from build123d import *

# Parameters (mm, degrees)
BOSS_EXTRUDE1_DEPTH = 3
BOSS_EXTRUDE2_DEPTH = 3
BOSS_EXTRUDE3_DEPTH = 30
FILLET1_R           = 3
CUT_EXTRUDE1_REACH  = 120.494
SKETCH6_R           = 7.5
CUT_EXTRUDE2_REACH  = 120.494
SKETCH7_W           = 30
SKETCH7_H           = 10
CUT_EXTRUDE3_START  = -36
SKETCH8_R           = 2.1
CUT_EXTRUDE3_DEPTH  = 36
FILLET2_R           = 1


with BuildPart() as part:
    # Sketch2 → Boss-Extrude1 (new body)
    with BuildSketch(Plane.XY):
        Polygon((165.715003736, 148.457007378), (35.636413421, 16.910208322), (54.124071667, -1.371107074), (184.202661981, 130.175691982), align=None)
    extrude(amount=-BOSS_EXTRUDE1_DEPTH)



with BuildPart() as body_2:
    # Sketch4 → Boss-Extrude2 (new body)
    with BuildSketch(Plane(origin=(0, 0, -36), x_dir=(-1, 0, 0), z_dir=(0, 0, -1))):
        Polygon((-165.715003736, 148.457007378), (-184.202661981, 130.175691982), (-54.124071667, -1.371107074), (-35.636413421, 16.910208322), align=None)
    extrude(amount=-BOSS_EXTRUDE2_DEPTH)


with BuildPart() as part_1:
    add(part.part)

    add(body_2.part)  # Boss-Extrude3 merges body 2
    # Sketch5 → Boss-Extrude3 (add)
    with BuildSketch(Plane(origin=(0, 0, -3), x_dir=(-1, 0, 0), z_dir=(0, 0, -1))):
        Polygon((-35.636413421, 16.910208322), (-165.715003736, 148.457007378), (-167.848195072, 146.347624832), (-37.769604757, 14.800825776), align=None)
    extrude(amount=BOSS_EXTRUDE3_DEPTH)

    # Fillet1
    fillet1_edges = [part_1.edges().sort_by_distance(p)[0] for p in [
        (100.675708579, 82.68360785, -36),
        (102.808899915, 80.574225304, -33),
        (102.808899915, 80.574225304, -3),
        (100.675708579, 82.68360785, 0),
    ]]
    fillet(fillet1_edges, radius=FILLET1_R)

    # Sketch6 → Cut-Extrude1 (cut, up to next)
    with BuildSketch(Plane(origin=(9.563615855, -9.456875254, 0), x_dir=(0, 0, 1), z_dir=(-0.711063779, 0.703127515, 0)), mode=Mode.PRIVATE) as cut_extrude1_sk1:
        with Locations((-18, 197.081179448)):
            Circle(SKETCH6_R)
    cut_extrude1_tool1 = extrude(cut_extrude1_sk1.sketch, amount=-CUT_EXTRUDE1_REACH, mode=Mode.PRIVATE) & part_1.part
    add(cut_extrude1_tool1.solids().sort_by_distance((148.136816, 130.680413, -18))[0], mode=Mode.SUBTRACT)

    # Sketch7 → Cut-Extrude2 (cut, up to next)
    with BuildSketch(Plane(origin=(9.563615855, -9.456875254, 0), x_dir=(0, 0, 1), z_dir=(-0.711063779, 0.703127515, 0)), mode=Mode.PRIVATE) as cut_extrude2_sk1:
        with Locations((-18, 217.081179448)):
            Rectangle(SKETCH7_W, SKETCH7_H)
    cut_extrude2_tool1 = extrude(cut_extrude2_sk1.sketch, amount=-CUT_EXTRUDE2_REACH, mode=Mode.PRIVATE) & part_1.part
    add(cut_extrude2_tool1.solids().sort_by_distance((162.199366, 144.901688, -18))[0], mode=Mode.SUBTRACT)
    # Sketch7 → Cut-Extrude2 (cut, up to next)
    with BuildSketch(Plane(origin=(9.563615855, -9.456875254, 0), x_dir=(0, 0, 1), z_dir=(-0.711063779, 0.703127515, 0)), mode=Mode.PRIVATE) as cut_extrude2_sk2:
        with Locations((-18, 42.081179448)):
            Rectangle(SKETCH7_W, SKETCH7_H)
    cut_extrude2_tool2 = extrude(cut_extrude2_sk2.sketch, amount=-CUT_EXTRUDE2_REACH, mode=Mode.PRIVATE) & part_1.part
    add(cut_extrude2_tool2.solids().sort_by_distance((39.152051, 20.465527, -18))[0], mode=Mode.SUBTRACT)

    # Sketch8 → Cut-Extrude3 (cut)
    with BuildSketch(Plane.XY.offset(CUT_EXTRUDE3_START)):
        with Locations((176.077014239, 129.069414997)):
            Circle(SKETCH8_R)
        with Locations((165.411057559, 139.616327725)):
            Circle(SKETCH8_R)
        with Locations((44.473124942, 17.313357792)):
            Circle(SKETCH8_R)
        with Locations((55.139081623, 6.766445064)):
            Circle(SKETCH8_R)
    extrude(amount=CUT_EXTRUDE3_DEPTH, mode=Mode.SUBTRACT)

    # Fillet2
    fillet2_edges = [part_1.edges().sort_by_distance(p)[0] for p in [
        (148.136815855, 130.680412911, -25.5),
        (150.270007192, 128.571030365, -25.5),
    ]]
    fillet(fillet2_edges, radius=FILLET2_R)


solid = part_1.part
Geometry: final body of the model. Coordinates: model frame, mm. A direction names the side the tool comes from. Coordinates: 2 decimals unless noted, no trailing zeros.
(1) First-contact query: pin 1 (1 mm diameter, centred on y = 54.5, z = -16, fed in from -X); pin 2 (12 mm diameter, centred on y = 127, z = -25, fed in from +X); pin 3 (4 mm diameter, centred on x = 156.5, z = -12, fed in from -Y); pin 4 (4 mm diameter, centred on x = 44.47, y = 17.31, fed in from -Z). Flat tips, straight axial feed; report the tip coordinate or a pass-through.
(2) Material intervals for probe 1 along Z at (x, y) = (130.5, 88.5); probe 2 along Y at (x, z) = (86, -2); probe 3 along Y at (x, z) = (117.5, -1.5), sorted ascending.
(3) Access query for faces 1 (the face through (102.61, 79.15, -32.1)), 2 (the face through (42.925, 18.733, -1.521)). Directions: +Z, -Z, +X, -X, +Y, -Y. A direction counts if a zero-diameter tool reaches every point of the face in a straight line with its end or side. Return the directions, or none.
(4) Draft query along X for faces 3 (the face through (111, 71, -33)), 4 (the face through (100, 82, -18)), 5 (the face through (174.53, 130.49, -1.52)), 6 (the face through (102.61, 79.15, -3.9)). Return one class per face: pulls with the +X half, pulls with the -X half, needs draft (parallel to the pull), parting line crosses it, or undercut.
Solution:
1. pin 1: stops at x = 72.31
1. pin 2: stops at x = 154.65
1. pin 3: stops at y = 132.85
1. pin 4: passes through
2. probe 1: z = -36 to -33, -3 to 0
2. probe 2: y = 30.86 to 67.6
2. probe 3: y = 62.72 to 99.13
3. face 1: +X, -Y
3. face 2: +Z, -Z
4. face 3: needs draft
4. face 4: pulls with the -X half
4. face 5: undercut
4. face 6: pulls with the +X half
